Source: three-view drawing plus pictorial views. Frame: mm from the lowest corner of the part. Give positions to 0.01 mm unless a question says otherwise; leave off trailing zeros. Write each loop counter-clockwise with the first axis right and the second up, starting at its lowest first coordinate (ties: lowest second). Pieces come first, ordered by that corner, then holes. Notation, with made-up numbers: M 33,88 L 68,88 A8 cw 68,97 Z; hole C -26,55 d11. An arc over 180 degrees is marked long. One line per question, with ' | ' between items.
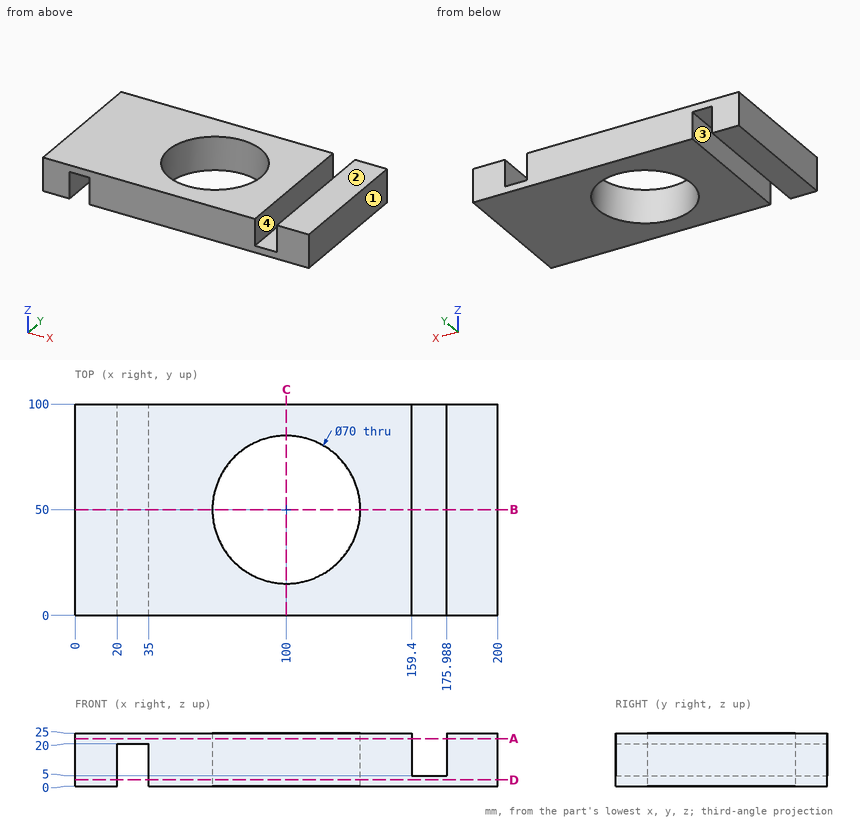
(1) Draft query along X for the marked faces 1, 2, 3 and 4. Return one class per face: released by +X, released by -X, zero draft, split by the parting line, or undercut.
Working result:
face 1: released by +X | face 2: zero draft | face 3: undercut | face 4: undercut
(2) Material intervals for L1, parallel to X at y = 48.5, z = 4.75; L2, parallel to X at y = 87, z = 10.25; L3, parallel to Y at x = 100, z = 10.25, sorted ascending. Write a range as [from, to].
Working result:
L1: x = [0, 20], [35, 65.03], [134.97, 200] | L2: x = [0, 20], [35, 159.4], [175.99, 200] | L3: y = [0, 15], [85, 100]
(3) First-contact query: P1, Ø1.5, axis at y = 59.5, z = 15, coming from the -X side; P2, Ø12, axis at x = 28.5, y = 46.5, coming from the -Z side. Flat tips, straight axial feed; report the tip coordinate or a pass-through.
Working result:
P1: stops at x = 0 | P2: stops at z = 20
(4) Cut plane A-A, the plane z = 22.5. Return loops of the section in (x, y).
Working result:
outline: M 0,0 L 159.4,0 L 159.4,100 L 0,100 Z; M 175.99,0 L 200,0 L 200,100 L 175.99,100 Z; hole C 100,50 d70
(5) Cut plane C-C, the plane x = 100. Return loops of the section in (y, z), then the cut area to 3 significant figures.
Working result:
outline: M 0,0 L 15,0 L 15,25 L 0,25 Z; M 85,0 L 100,0 L 100,25 L 85,25 Z | area: 750 mm^2
(6) Cut plane D-D, the plane z = 3. Return loops of the section in (x, y).
Working result:
outline: M 0,0 L 20,0 L 20,100 L 0,100 Z; M 35,0 L 200,0 L 200,100 L 35,100 Z; hole C 100,50 d70
(7) Cut plane B-B, the plane y = 50. Return loops of the section in (x, z).
Working result:
outline: M 0,0 L 20,0 L 20,20 L 35,20 L 35,0 L 65,0 L 65,25 L 0,25 Z; M 135,0 L 200,0 L 200,25 L 175.99,25 L 175.99,5 L 159.4,5 L 159.4,25 L 135,25 Z
